from build123d import *

# Parameters (mm, degrees)
CROQUIS1_R              = 1
SALIENTE_EXTRUIR1_DEPTH = 6
CROQUIS2_W              = 5
CROQUIS2_H              = 2
CORTAR_EXTRUIR1_DEPTH   = 8
REDONDEO1_R             = 4.5
REDONDEO2_R             = 3
CORTAR_EXTRUIR3_START   = -1
CORTAR_EXTRUIR3_DEPTH   = 1


with BuildPart() as part:
    # Croquis1 → Saliente-Extruir1 (new body)
    # profile 1 of 2: a face of its own
    with BuildSketch(Plane.XY):
        with BuildLine():
            Line((-0.968245837, -0.25), (-2.5, -0.25))
            ThreePointArc((-2.5, -0.25), (0, -2.75), (2.5, -0.25))
            Line((2.5, -0.25), (0.968245837, -0.25))
            ThreePointArc((0.968245837, -0.25), (0, -1), (-0.968245837, -0.25))
        make_face()
    # profile 2 of 2: a face of its own
    with BuildSketch(Plane.XY):
        with BuildLine():
            Line((-2.5, -0.25), (-0.968245837, -0.25))
            ThreePointArc((-0.968245837, -0.25), (0, 1), (0.968245837, -0.25))
            Line((0.968245837, -0.25), (2.5, -0.25))
            Line((2.5, -0.25), (2.5, 42))
            Line((2.5, 42), (-2.5, 42))
            Line((-2.5, 42), (-2.5, -0.25))
        make_face()
        with Locations((0, 38.5)):
            Circle(CROQUIS1_R, mode=Mode.SUBTRACT)
    extrude(amount=SALIENTE_EXTRUIR1_DEPTH)

    # Croquis2 → Cortar-Extruir1 (cut)
    with BuildSketch(Plane(origin=(0, 42, 0), x_dir=(1, 0, 0), z_dir=(0, 1, 0))):
        with Locations((0, -3)):
            Rectangle(CROQUIS2_W, CROQUIS2_H)
    extrude(amount=-CORTAR_EXTRUIR1_DEPTH, mode=Mode.SUBTRACT)

    # Redondeo1
    # the kernel refuses this fillet: 4.5 mm, written as the material it takes off along each edge
    with BuildSketch(Plane(origin=(-2.5, 34, 4), x_dir=(0, -1, 0), z_dir=(0, 0, -1)), Plane(origin=(2.5, 34, 2), x_dir=(0, -1, 0), z_dir=(0, 0, 1))) as redondeo1_piece_1:
        with BuildLine():
            CenterArc((REDONDEO1_R, -REDONDEO1_R), REDONDEO1_R, 90, 90)
            Line((0, -REDONDEO1_R), (0, 0))
            Line((0, 0), (REDONDEO1_R, 0))
        make_face()
    extrude(amount=2, mode=Mode.SUBTRACT)

    # Redondeo2
    # the kernel refuses this fillet: 3 mm, written as the material it takes off along each edge
    with BuildSketch(Plane(origin=(-2.5, 42, -3.5), x_dir=(0, -1, 0), z_dir=(0, 0, 1)), Plane(origin=(2.5, 42, -7.5), x_dir=(-1, 0, 0), z_dir=(0, 0, 1)), Plane(origin=(2.5, 42, -3.5), x_dir=(-1, 0, 0), z_dir=(0, 0, 1))) as redondeo2_piece_1:
        with BuildLine():
            CenterArc((REDONDEO2_R, REDONDEO2_R), REDONDEO2_R, 180, 90)
            Line((0, REDONDEO2_R), (0, 0))
            Line((0, 0), (REDONDEO2_R, 0))
        make_face()
    extrude(amount=17, mode=Mode.SUBTRACT)
    with BuildSketch(Plane(origin=(-2.5, 42, -7.5), x_dir=(1, 0, 0), z_dir=(0, 0, 1))) as redondeo2_piece_2:
        with BuildLine():
            CenterArc((REDONDEO2_R, -REDONDEO2_R), REDONDEO2_R, 90, 90)
            Line((0, -REDONDEO2_R), (0, 0))
            Line((0, 0), (REDONDEO2_R, 0))
        make_face()
    extrude(amount=17, mode=Mode.SUBTRACT)

    # Croquis4 → Cortar-Extruir3 (cut)
    with BuildSketch(Plane.XY.offset(6).offset(CORTAR_EXTRUIR3_START)):
        with BuildLine():
            Line((-2.5, 8.091687605), (-2.5, -0.25))
            ThreePointArc((-2.5, -0.25), (0, -2.75), (2.5, -0.25))
            Line((2.5, -0.25), (2.5, 8.091687605))
            ThreePointArc((2.5, 8.091687605), (0, 6.75), (-2.5, 8.091687605))
        make_face()
    cortar_extruir3 = extrude(amount=CORTAR_EXTRUIR3_DEPTH, mode=Mode.SUBTRACT)

    # Simetría1: Cortar-Extruir3 across plane
    add(cortar_extruir3.mirror(Plane.XY.offset(3)), mode=Mode.SUBTRACT)


solid = part.part
For this review, take the finished solid that the model builds, in its own axes (mm). A direction names the side the tool comes from. Give positions to 0.01 mm unless a question says otherwise; leave off trailing zeros. Order: outer loops, then holes, each group sorted by start corner. A loop starts at its lowest first (then second) coordinate and runs counter-clockwise, first axis right, second up. Notation, with made-up numbers: M -4,46.25 L 20,46.25 A25 ccw 20,59.25 Z; hole C 84,34.25 d8. An arc over 180 degrees is marked long. Answer in a Markdown table with one row per item. Add a question column.
(1) Consider section A-A on z = 4.4. State the section outline as (x, y) points.
(2) Consider section D-D on y = 4. State the section outline as (x, z) points.
(3) Wall thickness on probe 1 along X at (y, z) = (38.5, 1.1); probe 2 along Y at (x, z) = (0.2, 1.9); probe 3 along Z at (x, y) = (0.7, 33.5): over which ranges is each line inside the solid? List them lowest first. Write a range as [from, to].
(4) Consider section C-C on x = -0.5. State the section outline as (y, z) points, and give its area (3 significant figures).
(5) For pin 1 (1.5 mm diameter, centred on x = 1.5, z = 3.5, fed in from +Y); pin 2 (2.5 mm diameter, centred on x = -0.5, y = 4, fed in from +Z); pin 3 (1 mm diameter, centred on x = 2, z = 2, fed in from +Y), all flat-tipped, find the tip position at first contact; note any pin that passes through.
(6) Consider section B-B on y = 38. State the section outline as (x, z) points, and give its area (3 significant figures).
(7) Mouldability with a two-part tool opening along Y and no side actions: class faces 6 (the face through (-0.05, -2.75, 2.97)), 7 (the face through (0, 25, 0)), 8 (the face through (-0.13, 39.49, 0.99)) as +Y half, -Y half, draft (parallel to the pull), parting line (faces both ways), or undercut.
(8) For faces 1 (the face through (-1.77, 40.96, 4.99)), 2 (the face through (1.843, 31.842, 2.986)), 3 (the face through (2.5, 19, 3)), 4 (the face through (0.04, 6.75, 0.51)), 5 (the face through (-1.843, 31.842, 3.014)), list the 3-axis set-ups (+Z, -Z, +X, -X, +Y, -Y) from which the entire face can be reached by the end or side of a thin tool; tool diameter is ignored.
Evaluation:
| question | item | result |
|---|---|---|
| 1 | outline | M -2.5,-0.25 A2.5 ccw 2.5,-0.25 L 2.5,39 A3 ccw 0,41.96 A3 ccw -2.5,39 Z; hole C 0,0 d2; hole C 0,38.5 d2 |
| 2 | outline | M -2.5,1 L 2.5,1 L 2.5,5 L -2.5,5 Z |
| 3 | probe 1 | x = [-2.5, -1], [1, 2.5] |
| 3 | probe 2 | y = [-2.74, -0.98], [0.98, 37.52], [39.48, 41.92] |
| 3 | probe 3 | z = [0, 2], [4, 6] |
| 4 | outline | M -2.7,1 L -0.87,1 L -0.87,5 L -2.7,5 Z; M 0.87,1 L 6.79,1 L 6.79,0 L 37.63,0 L 37.63,2 L 33.24,2 L 33.24,4 L 37.63,4 L 37.63,6 L 6.79,6 L 6.79,5 L 0.87,5 Z; M 39.37,0 L 41.83,0 L 41.83,2 L 39.37,2 Z; M 39.37,4 L 41.83,4 L 41.83,6 L 39.37,6 Z |
| 4 | area | 217 mm^2 |
| 5 | pin 1 | stops at y = 41.63 |
| 5 | pin 2 | stops at z = 5 |
| 5 | pin 3 | stops at y = 41.24 |
| 6 | outline | M -2.5,0 L -0.87,0 L -0.87,2 L -2.5,2 Z; M -2.5,4 L -0.87,4 L -0.87,6 L -2.5,6 Z; M 0.87,0 L 2.5,0 L 2.5,2 L 0.87,2 Z; M 0.87,4 L 2.5,4 L 2.5,6 L 0.87,6 Z |
| 6 | area | 13.1 mm^2 |
| 7 | face 6 | -Y half |
| 7 | face 7 | draft |
| 7 | face 8 | undercut |
| 8 | face 1 | +Z, -Z, -X, +Y |
| 8 | face 2 | +X, +Y |
| 8 | face 3 | +Z, -Z, +X, +Y, -Y |
| 8 | face 4 | -Z, -Y |
| 8 | face 5 | -X, +Y |
